Can you work these out from the model? Positions are in its coordinate system, mm. A direction names the side the tool comes from. Round coordinates to 2 decimals unless told otherwise and drop trailing zeros. Write each loop counter-clockwise with the first axis right and the second up, starting at its lowest first coordinate (ties: lowest second). Pieces come first, ordered by that corner, then holes.
Q1. If we section it at C-C (x = -83.5): Please give me the cut outline in (y, z) (3 decimals), plus the area to 3 significant figures.
Q2. For faces 4 (the cylindrical face through (21.74, 12.34, 7.44)), 5 (the cylindrical face through (-21.2, -2.4, 10)), 6 (the flat face through (-82, 38, 15)), 7 (the flat face through (-12, 4, 3.5)), which set-ups out of +Z, -Z, +X, -X, +Y, -Y let a thin tool reach every point of the face, with its end or its side?
Q3. Please list where these lines run through material, in increasing order: line 1 along Y through (x, z) = (0, 10.15); line 2 along X through (y, z) = (-5.5, 4.75); line 3 along X through (y, z) = (-18, 5.25).
Q4. If we section it at B-B (y = 58): Please give me the cut outline in (x, z), plus the area to 3 significant figures.
Q5. We'd pull the mould along X, two halves only. Please class faces 1 (the cylindrical face through (95.38, 30.04, 7.4)), 2 (the flat face through (-82, 38, 0)), 3 (the flat face through (-6.4, 9.4, 11.5)): +X half, -X half, draft (parallel to the pull), parting line (faces both ways), or undercut.
Q6. If we section it at D-D (z = 5.75): Give the number of separate pieces and of enclosed holes in the cut face, plus the area to 3 significant figures.
Q7. If we section it at A-A (x = -49): Please give me the cut outline in (y, z).
Q8. I'm going to push flat-ended pins straight in: pin 1 Ø4 at (x, y) = (1.5, -18) entering from +Z; pin 2 Ø3 at (y, z) = (-79, 4.5) entering from +X; pin 3 Ø4 at (x, y) = (-66.5, -78) entering from +Z; pin 4 Ø10.5 at (x, y) = (-18, 0) entering from +Z. Where does each tip first touch, or does it pass through?
from build123d import *

# Parameters (mm, degrees)
SKETCH1_R               = 100
BOSS_EXTRUDE1_DEPTH     = 15
CUT_EXTRUDE1_DEPTH      = 143.214626533
CUT_EXTRUDE1_DEPTH_BACK = 143.214626533
SKETCH2_R               = 90
BOSS_EXTRUDE3_START     = 3.5
SKETCH5_R               = 25
BOSS_EXTRUDE3_DEPTH     = 8
BOSS_EXTRUDE4_START     = 3.5
SKETCH6_W               = 14
SKETCH6_H               = 70
BOSS_EXTRUDE4_DEPTH     = 8
SKETCH9_R               = 11.1
CUT_EXTRUDE4_DEPTH      = 143.214626533
SKETCH10_R              = 2.05
CUT_EXTRUDE5_DEPTH      = 143.214626533
FILLET3_R               = 10
CUT_EXTRUDE6_START      = 8.5
SKETCH11_R              = 4
CUT_EXTRUDE6_DEPTH      = 3


with BuildPart() as part:
    # Sketch1 → Boss-Extrude1 (new body)
    with BuildSketch(Plane.XY):
        Circle(SKETCH1_R)
    extrude(amount=BOSS_EXTRUDE1_DEPTH)

    # Sketch2 → Cut-Extrude1 (cut, two sides: drawn at the far end of the back side and taken through both)
    with BuildSketch(Plane.XY.offset(-CUT_EXTRUDE1_DEPTH_BACK)):
        Circle(SKETCH2_R)
    extrude(amount=CUT_EXTRUDE1_DEPTH + CUT_EXTRUDE1_DEPTH_BACK, mode=Mode.SUBTRACT)



with BuildPart() as body_2:
    # Sketch5 → Boss-Extrude3 (new body)
    with BuildSketch(Plane.XY.offset(BOSS_EXTRUDE3_START)):
        Circle(SKETCH5_R)
    extrude(amount=BOSS_EXTRUDE3_DEPTH)


with BuildPart() as part_1:
    add(part.part)

    add(body_2.part)  # Boss-Extrude4 merges body 2
    # Sketch6 → Boss-Extrude4 (add)
    with BuildSketch(Plane.XY.offset(BOSS_EXTRUDE4_START)):
        with Locations((0, 59)):
            Rectangle(SKETCH6_W, SKETCH6_H)
        Polygon((17.284609691, -18.062177826), (77.906387956, -53.062177826), (84.906387956, -40.937822174), (24.284609691, -5.937822174), align=None)
        Polygon((-17.284609691, -18.062177826), (-77.906387956, -53.062177826), (-84.906387956, -40.937822174), (-24.284609691, -5.937822174), align=None)
    extrude(amount=BOSS_EXTRUDE4_DEPTH)

    # Sketch9 → Cut-Extrude4 (cut, through all)
    with BuildSketch(Plane.XY):
        Circle(SKETCH9_R)
    extrude(amount=CUT_EXTRUDE4_DEPTH, mode=Mode.SUBTRACT)

    # Sketch10 → Cut-Extrude5 (cut, through all)
    with BuildSketch(Plane.XY):
        with Locations((0, 18)):
            Circle(SKETCH10_R)
        with Locations((18, 0)):
            Circle(SKETCH10_R)
        with Locations((0, -18)):
            Circle(SKETCH10_R)
        with Locations((-18, 0)):
            Circle(SKETCH10_R)
    extrude(amount=CUT_EXTRUDE5_DEPTH, mode=Mode.SUBTRACT)

    # Fillet3
    fillet3_edges = [part_1.edges().sort_by_distance(p)[0] for p in [
        (-7, 24, 7.5),
        (7, 24, 7.5),
        (24.284609691, -5.937822174, 7.5),
        (17.284609691, -18.062177826, 7.5),
        (-17.284609691, -18.062177826, 7.5),
        (-24.284609691, -5.937822174, 7.5),
    ]]
    fillet(fillet3_edges, radius=FILLET3_R)

    # Sketch11 → Cut-Extrude6 (cut)
    with BuildSketch(Plane.XY.offset(CUT_EXTRUDE6_START)):
        with Locations((18, 0)):
            Circle(SKETCH11_R)
        with Locations((0, -18)):
            Circle(SKETCH11_R)
        with Locations((-18, 0)):
            Circle(SKETCH11_R)
        with Locations((0, 18)):
            Circle(SKETCH11_R)
    extrude(amount=CUT_EXTRUDE6_DEPTH, mode=Mode.SUBTRACT)


solid = part_1.part
A:
1. outline: (-55.025, 0) - (-33.582, 0) - (-33.582, 15) - (-55.025, 15) - close; (33.582, 0) - (55.025, 0) - (55.025, 15) - (33.582, 15) - close
1. area: 643 mm2
2. face 4: +Z, -Z
2. face 5: +Z
2. face 6: +Z, +X, -X, +Y, -Y
2. face 7: -Z
3. line 1: y = -100 to -90, -25 to -22, -14 to -11.1, 11.1 to 14, 22 to 100
3. line 2: x = -99.85 to -89.83, -26.29 to -9.64, 9.64 to 26.29, 89.83 to 99.85
3. line 3: x = -98.37 to -88.18, -45.18 to -2.05, 2.05 to 45.18, 88.18 to 98.37
4. outline: (-81.46, 0) - (-68.82, 0) - (-68.82, 15) - (-81.46, 15) - close; (-7, 3.5) - (7, 3.5) - (7, 11.5) - (-7, 11.5) - close; (68.82, 0) - (81.46, 0) - (81.46, 15) - (68.82, 15) - close
4. area: 491 mm2
5. face 1: parting line
5. face 2: draft
5. face 3: undercut
6. separate pieces: 1
6. enclosed holes: 8
6. area: 10,300 mm2
7. outline: (-87.17, 0) - (-75.49, 0) - (-75.49, 15) - (-87.17, 15) - close; (-36.37, 3.5) - (-20.21, 3.5) - (-20.21, 11.5) - (-36.37, 11.5) - close; (75.49, 0) - (87.17, 0) - (87.17, 15) - (75.49, 15) - close
8. pin 1: stops at z = 8.5
8. pin 2: stops at x = 63.2
8. pin 3: passes through
8. pin 4: stops at z = 11.5
